Autodesk Inventor part; units mm, degrees
ref_plane "YZ Plane" through (0, 0, 0) normal (1, 0, 0) x (0, 1, 0)
ref_plane "XZ Plane" through (0, 0, 0) normal (0, 1, 0) x (-1, 0, 0)
ref_plane "XY Plane" through (0, 0, 0) normal (0, 0, 1) x (1, 0, 0)
sketch "Boceto9" plane through (0, 0, 0) normal (1, 0, 0) x (0, 1, 0)
  line L0 (0, 0) -> (0, -3)
  line L1 (0, -3) -> (0, -33)
  line L2 (0, -3) -> (3, -3)
  line L3 (3, -3) -> (3, -33)
  line L4 (3, -33) -> (0, -33)
  line L5 (3, -3) -> (3, -18)
  line L6 (3, -18) -> (7.8231, 0)
  line L7 (7.8231, 0) -> (0, 0)
  dimension "d22" = 3
  dimension "d23" = 30
  dimension "d24" = 3
  dimension "d25" = 15
  dimension "d26" = 15
extrude "Extrusión6" add sketch "Boceto9" along normal blind 22
sketch "Boceto10" plane through (0, 0, -33) normal (0, -1, 0) x (1, 0, 0)
  line L0 (22, 15) -> (22, 33)
  line L1 (22, 33) -> (22, 30)
  line L2 (22, 30) -> (22.6923, 30)
  line L3 (22, 30) -> (32, 30)
  line L4 (32, 30) -> (32, 3)
  line L5 (32, 3) -> (22, 3)
  line L6 (22, 0) -> (22, 15)
  line L7 (0, 33) -> (22, 33)
  line L8 (11, 33) -> (11, 0)
  line L9 (0, 0) -> (22, 0)
  line L10 (0, 15) -> (0, 33)
  line L11 (0, 33) -> (0, 30)
  line L12 (0, 30) -> (-0.6923, 30)
  line L13 (0, 30) -> (-10, 30)
  line L14 (-10, 30) -> (-10, 3)
  line L15 (-10, 3) -> (0, 3)
  line L16 (0, 0) -> (0, 15)
  line L17 (22, 33) -> (0, 33)
  line L18 (22, 0) -> (0, 0)
  dimension "d29" = 3
  dimension "d31" = 10
  dimension "d32" = 27
extrude "Extrusión7" add sketch "Boceto10" against normal blind 5 contours L0 L2 L3 L4 L5 L6 | L10 L16 L15 L14 L13 L12
sketch "Boceto11" plane through (32, 0, -3) normal (1, 0, 0) x (0, 0, -1)
  line L0 (27, 3) -> (15, 3)
  line L1 (15, 3) -> (7.5359, 5)
  line L2 (27, 5) -> (7.5359, 5)
  line L3 (27, 3) -> (15, 3)
  line L4 (15, 3) -> (7.5359, 5)
  line L5 (27, 5) -> (7.5359, 5)
  line L6 (27, 3) -> (27, 5)
  line L7 (27, 0) -> (0, 0)
  line L8 (0, 5) -> (27, 5)
  line L9 (0, 5) -> (27, 5)
  line L10 (27, 5) -> (7.5359, 5)
  line L11 (0, 5) -> (7.5359, 5)
  line L12 (27, 0) -> (0, 0)
  line L13 (27, 0) -> (27, 5)
  line L14 (0, 5) -> (27, 5)
  line L15 (0, 0) -> (0, 5)
  line L16 (27, 0) -> (30, 0)
  line L17 (30, 0) -> (30, 3)
  line L18 (27, 0) -> (27, 3)
  line L19 (30, 3) -> (27, 3)
  line L20 (30, 0) -> (30, 3)
  line L21 (27, 0) -> (30, 0)
  line L22 (30, 0) -> (30, 3)
  line L23 (30, 0) -> (30, 3)
  line L24 (30, 3) -> (27, 3)
  line L25 (30, 3) -> (27, 3)
  line L26 (27, 3) -> (15, 3)
  line L27 (27, 3) -> (15, 3)
  line L28 (30, 3) -> (27, 3)
  line L29 (-3, 0) -> (0, 0)
  line L30 (0, 0) -> (27, 0)
  line L31 (27, 0) -> (30, 0)
  line L32 (27, 0) -> (30, 0)
  line L33 (27, 0) -> (0, 0)
  line L34 (-3, 0) -> (0, 0)
  line L35 (15, 3) -> (7.5359, 5)
  line L36 (7.5359, 5) -> (-3, 7.8231)
  line L37 (7.5359, 5) -> (-3, 7.8231)
  line L38 (15, 3) -> (7.5359, 5)
  line L39 (27, 0) -> (27, 3)
  line L40 (27, 0) -> (27, 5)
  line L41 (15, 3) -> (7.5359, 5)
  line L42 (7.5359, 5) -> (27, 5)
  line L43 (27, 3) -> (27, 5)
  line L44 (27, 3) -> (15, 3)
  line L45 (27, 3) -> (15, 3)
  line L46 (27, 3) -> (27, 5)
  line L47 (7.5359, 5) -> (27, 5)
  line L48 (15, 3) -> (7.5359, 5)
  line L49 (27, 0) -> (27, 5)
  line L50 (27, 3) -> (27, 5)
  line L51 (27, 0) -> (27, 3)
  line L52 (27, 5) -> (0, 5)
  line L53 (7.5359, 5) -> (0, 5)
  line L54 (7.5359, 5) -> (27, 5)
  line L55 (0, 0) -> (27, 0)
  line L56 (0, 0) -> (0, 5)
  line L57 (27, 5) -> (0, 5)
  line L58 (27, 0) -> (27, 5)
  line L59 (0, 0) -> (27, 0)
  line L60 (27, 5) -> (0, 5)
  line L61 (27, 3) -> (27, 0)
  line L62 (27, 3) -> (27, 5)
  line L63 (30, 3) -> (27, 3)
  line L64 (30, 0) -> (30, 3)
  line L65 (27, 0) -> (30, 0)
  line L66 (27, 0) -> (27, 5)
  line L67 (27, 3) -> (27, 0)
  line L68 (27, 3) -> (27, 5)
  line L69 (27, 0) -> (27, 5)
  line L70 (27, 3) -> (27, 0)
  line L71 (27, 0) -> (30, 0)
  line L72 (30, 0) -> (30, 3)
  line L73 (30, 3) -> (27, 3)
extrude "Extrusión8" cut sketch "Boceto11" against normal up to surface (42 mm away) contours L0 L1 L2 L6
sketch "Boceto12" plane through (22, 0, 0) normal (1, 0, 0) x (0, 0, -1)
  line L0 (10.5359, 5) -> (0, 7.8231)
  line L1 (0, 7.8231) -> (5.1764, 27.1416)
  line L2 (0, 7.8231) -> (20, 7.8231) construction
  line L3 (5.1764, 27.1416) -> (13.8697, 24.8122)
  line L4 (13.8697, 24.8122) -> (8.6933, 5.4937)
  point P0 (0, 0)
  dimension "d37" = 20
  dimension "d38" = 75
  dimension "d40" = 9
extrude "Extrusión9" add sketch "Boceto12" against normal up to surface (22 mm away)
sketch "Boceto13" plane through (22, 24.8122, -13.8697) normal (0, -0.2588, -0.9659) x (-1, 0, 0)
  line L0 (22, -20) -> (0, -20)
  line L1 (0, -20) -> (3, -20)
  line L2 (0, 0) -> (0, -20)
  line L3 (0, 0) -> (3, 0)
  line L4 (0, 0) -> (22, 0)
  line L5 (3, 0) -> (3, -16.1177)
  line L6 (0, 0) -> (0, -3)
  line L7 (0, -3) -> (22, -3)
  line L8 (22, -3) -> (22, 0)
  line L9 (22, 0) -> (19, 0)
  line L10 (19, 0) -> (19, -20)
  line L11 (3, -3) -> (3, -20)
  point P0 (22, -27.5565)
  point P1 (19, -3)
  dimension "d43" = 3
  dimension "d44" = 3
  dimension "d45" = 3
  dimension "d46" = 3
extrude "Extrusión10" cut sketch "Boceto13" against normal blind 7 contours L0 L11 L5 L7 L10
sketch "Boceto14" plane through (0, 0, -33) normal (0, -1, 0) x (1, 0, 0)
  line L0 (32, 30) -> (32, 22.4641)
  line L1 (32, 30) -> (32, 27)
  line L2 (32, 30) -> (29, 30)
  line L3 (22, 30) -> (32, 30)
  line L4 (29, 30) -> (29, 3)
  line L5 (32, 3) -> (32, 30)
  line L6 (29, 3) -> (32, 3)
  line L7 (32, 3) -> (32, 6)
  line L8 (32, 6) -> (25, 6)
  line L9 (25, 6) -> (22, 6)
  line L10 (22, 6) -> (22, 30)
  line L11 (22, 30) -> (22, 27)
  line L12 (22, 27) -> (32, 27)
  line L13 (22, 3) -> (25, 3)
  line L14 (25, 3) -> (25, 30)
  line L15 (29, 27) -> (27.5, 27)
  line L16 (27.5, 27) -> (27.5, 6)
  line L17 (27.5, 6) -> (29, 6)
  line L18 (29, 6) -> (29, 27)
  line L19 (25, 27) -> (26.5, 27)
  line L20 (26.5, 27) -> (26.5, 6)
  line L21 (26.5, 6) -> (25, 6)
  line L22 (25, 6) -> (25, 27)
  line L23 (0, 33) -> (22, 33)
  line L24 (11, 33) -> (11, -0.1638)
  line L25 (-10, 30) -> (-10, 22.4641)
  line L26 (-10, 30) -> (-10, 27)
  line L27 (-10, 30) -> (-7, 30)
  line L28 (0, 30) -> (-10, 30)
  line L29 (-7, 30) -> (-7, 3)
  line L30 (-10, 3) -> (-10, 30)
  line L31 (-7, 3) -> (-10, 3)
  line L32 (-10, 3) -> (-10, 6)
  line L33 (-10, 6) -> (-3, 6)
  line L34 (-3, 6) -> (0, 6)
  line L35 (0, 6) -> (0, 30)
  line L36 (0, 30) -> (0, 27)
  line L37 (0, 27) -> (-10, 27)
  line L38 (0, 3) -> (-3, 3)
  line L39 (-3, 3) -> (-3, 30)
  line L40 (-7, 27) -> (-5.5, 27)
  line L41 (-5.5, 27) -> (-5.5, 6)
  line L42 (-5.5, 6) -> (-7, 6)
  line L43 (-7, 6) -> (-7, 27)
  line L44 (-3, 27) -> (-4.5, 27)
  line L45 (-4.5, 27) -> (-4.5, 6)
  line L46 (-4.5, 6) -> (-3, 6)
  line L47 (-3, 6) -> (-3, 27)
  line L48 (22, 33) -> (0, 33)
  point P0 (-7, 6)
  point P1 (25, 6)
  point P2 (29, 6)
  dimension "d52" = 3
  dimension "d53" = 3
  dimension "d54" = 3
  dimension "d55" = 7
  dimension "d56" = 90
  dimension "d57" = 3
  dimension "d58" = 3
  dimension "d59" = 3
  dimension "d60" = 1.5
  dimension "d61" = 1.5
  dimension "d62" = 21
extrude "Extrusión11" cut sketch "Boceto14" against normal blind 7 contours L4 L8 L16 L12 | L12 L20 L8 L14 | L37 L41 L33 L29 | L39 L33 L45 L37
sketch "Boceto15" plane through (22, 26.624, -7.1082) normal (0, -0.2588, -0.9659) x (-1, 0, 0)
  line L0 (19, -20) -> (3, -20)
  line L1 (19, -3) -> (19, -20)
  line L2 (3, -3) -> (19, -3)
  line L3 (3, -20) -> (3, -3)
  line L4 (22, -19.0155) -> (0, -19.0155)
  line L5 (3, -20) -> (19, -20)
  line L6 (25, -20) -> (-3, -20)
  line L7 (3, -20) -> (11, -20)
  line L8 (3, -20) -> (19, -20)
  line L9 (11, -20) -> (11, -3)
  line L10 (11, -20) -> (11, -11.5)
  circle A0 centre (11, -11.5) radius 4.1
  point P0 (22, -27.5565)
  dimension "d65" = 8.5
  dimension "d66" = 8.2
extrude "Extrusión12" cut sketch "Boceto15" against normal blind 2 contours A0 L9 | L9 A0
sketch "Boceto17" plane through (22, 24.8122, -13.8697) normal (0, -0.2588, -0.9659) x (-1, 0, 0)
  line L0 (0, 0) -> (1.5, 0)
  line L1 (0, 0) -> (22, 0)
  line L2 (1.5, 0) -> (1.5, -1.5)
  line L3 (22, 0) -> (20.5, 0)
  line L4 (20.5, 0) -> (20.5, -1.5)
  line L5 (0, -20) -> (1.5, -20)
  line L6 (3, -20) -> (0, -20)
  line L7 (1.5, -20) -> (1.5, -18.5)
  line L8 (1.5, -18.5) -> (20.5, -18.5)
  circle A0 centre (1.5, -18.5) radius 0.75
  circle A1 centre (20.5, -18.5) radius 0.75
  circle A2 centre (20.5, -1.5) radius 0.75
  circle A3 centre (1.5, -1.5) radius 0.75
  point P0 (22, -27.5565)
  dimension "d69" = 1.5
  dimension "d70" = 1.5
  dimension "d71" = 1.5
  dimension "d72" = 1.5
  dimension "d73" = 1.5
  dimension "d74" = 1.5
  dimension "d75" = 19
  dimension "d76" = 1.5
  dimension "d77" = 1.5
  dimension "d78" = 1.5
  dimension "d79" = 1.5
extrude "Extrusión13" cut sketch "Boceto17" against normal blind 2
sketch "Boceto18" plane through (3, 7.3054, -1.9319) normal (0, 0.9659, -0.2588) x (1, 0, 0)
  line L0 (19, 8.9076) -> (19, 7)
  line L1 (19, 8.9076) -> (19, 16.635)
  line L2 (-6, 16.635) -> (22, 16.635)
  line L3 (19, 16.635) -> (-3, 16.635)
  line L4 (-3, 16.635) -> (8, 16.635)
  line L5 (8, 16.635) -> (6, 16.635)
  line L6 (6, 16.635) -> (10, 16.635)
  line L7 (10, 16.635) -> (10, 0.0248)
  line L8 (10, 0.0248) -> (6, 0.0248)
  line L9 (6, 0.0248) -> (6, 16.635)
  point P0 (-3, 0.0248)
  dimension "d82" = 2
  dimension "d83" = 4
  dimension "d84" = 4
extrude "Extrusión14" cut sketch "Boceto18" against normal blind 1
sketch "Boceto19" plane through (0, 3, -33) normal (0, 1, 0) x (1, 0, 0)
  line L0 (0, 0) -> (22, 0)
  line L1 (9, -15) -> (9, 0)
  line L2 (9, 0) -> (13, 0)
  line L3 (13, 0) -> (13, -15)
  line L4 (13, -15) -> (25, -15)
  line L5 (13, -15) -> (13, -17.039)
  line L6 (13, -15) -> (13, -31.0442)
  line L7 (9, -31.303) -> (9, -15.2588)
  line L8 (9, -17.039) -> (13, -17.039)
  line L9 (9, -17.039) -> (9, -14.1278)
  point P0 (0, -33)
  dimension "d87" = 4
extrude "Extrusión16" cut sketch "Boceto19" against normal blind 1
sketch "Boceto20" plane through (0, 0, -33) normal (0, 0, -1) x (-1, 0, 0)
  line L0 (-13, 2) -> (-9, 2)
  line L1 (-11, 2) -> (-9, 2)
  line L2 (-13, 2) -> (-13, 3)
  line L3 (-13, 3) -> (-11, 3)
  circle A0 centre (-11, 3) radius 3
  circle A1 centre (-11, 3) radius 2
  line L4 (-13, 3) -> (-22, 3)
  line L5 (-14.8156, 3) -> (-7.3833, 3)
  point P0 (0, 0)
  point P1 (-8, 3)
  point P2 (-9, 3)
  point P3 (-12.7321, 2)
  point P4 (-14, 3)
  dimension "d92" = 2
  dimension "d93" = 6
  dimension "d94" = 4
extrude "Extrusión17" add sketch "Boceto20" along normal blind 20 contours L0 A1 L5 A0 L4 L2
properties part number "pieza prueba autodesk"
Verification items for the finished model (mm, model axes). A direction names the side the tool comes from. Coordinates: 2 decimals unless noted, no trailing zeros. Write each loop counter-clockwise with the first axis right and the second up, starting at its lowest first coordinate (ties: lowest second). Pieces come first, ordered by that corner, then holes. Notation, with made-up numbers: (-25.75, 37) - (27.25, 37) arc R19 ccw to (27.25, 41) - close; hole circle Ø1 at (31, 86). An arc over 180 degrees is marked (long way). Write item = value, one per line.
Q1. Cross-section at D-D (z = -40). Enter the section's corners in (x, y), plus the area to 3 significant figures.
Answer:
outline = (8, 3) arc R3 ccw to (14, 3) - (13, 3) - (13, 2) - (12.73, 2) arc R2 cw to (9, 3) - close
area = 7.77 mm²
Q2. Material ranges on L1, parallel to Y at x = -2, z = -28; L2, parallel to Y at x = 12.5, z = -30.5; L3, parallel to Y at x = 13.5, z = -8 (3 decimals), recorded low to high. Write a range as from..to.
Answer:
L1 = 0..3
L2 = 0..2
L3 = 0..5.679, 23.279..26.385
Q3. Cross-section at C-C (y = 10.5). Enter the section's corners in (x, z), plus the area to 3 significant figures.
Answer:
outline = (0, -10.03) - (3, -10.03) - (3, -2.79) - (19, -2.79) - (19, -10.03) - (22, -10.03) - (22, -0.72) - (0, -0.72) - close
area = 89.0 mm²
Q4. Access from +Z, -Z, +X, -X, +Y, -Y to the whole of each face (thin tool, end or side, straight path). Record for faces 5 (the face through (-5, 1, -30)), 6 (the face through (11, 4, 0)), 7 (the face through (20, 3, -27)), 8 (the face through (7.213, 14.254, -2.772)), 9 (the face through (-4.5, 2, -14)).
Answer:
face_5 = -Z, -X, +Y, -Y
face_6 = +Z, +X, -X, +Y, -Y
face_7 = -Z, +X, -X, +Y
face_8 = none
face_9 = +Y, -Y
Q5. Go/stop test with flat-tipped pins: pin 1 Ø4 at (x, z) = (-2, -25.5) entering from +Y; pin 2 Ø8 at (x, y) = (23, 22.5) entering from +Z; pin 3 Ø4 at (x, z) = (29, -6) entering from +Y; pin 4 Ø1.6 at (y, z) = (4.5, -22) entering from -X. Record where each tip stops, or that it passes through.
Answer:
pin_1 = 3
pin_2 = -2.89
pin_3 = 5
pin_4 = through
Q6. Mould release check, pull along Y, two halves, no side actions. Record for faces 1 (the face through (13, 2.5, -27.2)), 2 (the face through (22, 14, -7)), 3 (the face through (27, 5, -7)), 4 (the face through (12.89, 19.28, -5.14)): released by +Y, released by -Y, zero draft, split by the parting line, or undercut.
Answer:
face_1 = undercut
face_2 = zero draft
face_3 = released by +Y
face_4 = undercut
Q7. Cross-section at B-B (x = 6). Enter the section's corners in (y, z), plus the area to 3 significant figures.
Answer:
outline = (0, -33) - (3, -33) - (3, -18) - (5.49, -8.69) - (7.31, -1.93) - (23.73, -6.33) - (21.91, -13.09) - (24.81, -13.87) - (27.14, -5.18) - (7.82, 0) - (0, 0) - close
area = 203 mm²
Q8. Cross-section at A-A (z = -28). Enter the section's corners in (x, y), plus the area to 3 significant figures.
Answer:
outline = (-10, 0) - (32, 0) - (32, 3) - (13, 3) - (13, 2) - (9, 2) - (9, 3) - (-10, 3) - close
area = 122 mm²
